Read the model definition and answer for the solid it produces. Units are mm, in the model's axes. Face numbers are marked on the shaded views. A direction names the side the tool comes from. Coordinates: 2 decimals unless noted, no trailing zeros. Order: outer loops, then holes, each group sorted by start corner. A loop starts at its lowest first (then second) coordinate and runs counter-clockwise, first axis right, second up. Notation, with made-up numbers: M -5,-29.75 L 42,-29.75 A22 cw 42,-12.75 Z; hole C 43.5,49 d6. An arc over 180 degrees is marked long. One line per question, with ' | ' between items. Start each with the question number.
1) Find section A-A, the plane z = 20. Write down the section's boundary in (x, y), plus the area to 3 significant figures.
2) Find section B-B, the plane x = 136. Write down the section's boundary in (y, z), plus the area to 3 significant figures.
3) A tool of negligible diameter and unlimited length cuts with its end or side. For the marked faces 1 and 2, from which of +Z, -Z, +X, -X, +Y, -Y can it reach the whole face along a straight path? Write none if from no direction.
4) Given P1, Ø5, axis at x = 72.5, y = 251.5, coming from the +Z side; P2, Ø5, axis at x = 79, z = 17, coming from the -Y side; P3, Ø5.5, axis at x = 76.2, z = 88.9, coming from the -Y side, each flat-ended and moving along its own axis, determine where each tip first touches the part or whether it passes through.
5) Consider probe 1 along Y at (x, z) = (77.5, 151); probe 2 along Z at (x, y) = (76, 8). Determine where each line is inside the solid, lowest interval first.
6) Find section C-C, the plane y = 323.5. Write down the section's boundary in (x, z), plus the area to 3 significant figures.
7) Find section D-D, the plane z = 122. Write down the section's boundary in (x, y), plus the area to 3 significant figures.
8) The mould has two halves that part along Y. Classify the marked faces 3, 4 and 5: +Y half, -Y half, draft (parallel to the pull), parting line (faces both ways), or undercut.
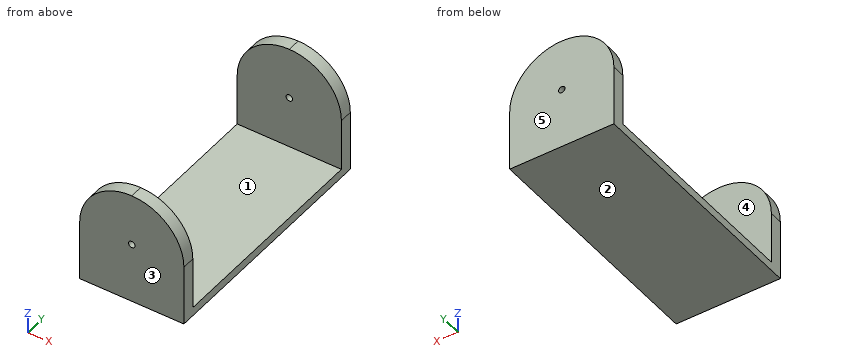
from build123d import *

# Parameters (mm, degrees)
F0_W     = 19.05
F0_H     = 152.4
F0_H_2   = 12.7
F0_W_2   = 317.5
F1_DEPTH = 152.4
F2_R     = 4.7625
F3_DEPTH = 406.4
F4_R     = 76.19999


# Not quite as in the source:
# - a fillet or chamfer is up to 0.001 mm smaller than in the source, because OpenCascade refuses the exact size


with BuildPart() as f1:
    # F0 (on Right) → F1 (new body)
    with BuildSketch(Plane.YZ):
        with Locations((9.525, 88.9)):
            Rectangle(F0_W, F0_H)
        with Locations((9.525, 6.35)):
            Rectangle(F0_W, F0_H_2)
        with Locations((177.8, 6.35)):
            Rectangle(F0_W_2, F0_H_2)
        with Locations((346.075, 88.9)):
            Rectangle(F0_W, F0_H)
        with Locations((346.075, 6.35)):
            Rectangle(F0_W, F0_H_2)
    extrude(amount=F1_DEPTH)

    # F2 (on Front) → F3 (cut)
    with BuildSketch(Plane.XZ):
        with Locations((76.2, 88.9)):
            Circle(F2_R)
    extrude(amount=-F3_DEPTH, mode=Mode.SUBTRACT)

    # F4 (radius 76.2 in the source; OpenCascade refuses exactly that, so slightly less here)
    f4_edges = [f1.edges().sort_by_distance(p)[0] for p in [
        (152.4, 346.075, 165.1),
        (152.4, 9.525, 165.1),
        (0, 9.525, 165.1),
        (0, 346.075, 165.1),
    ]]
    fillet(f4_edges, radius=F4_R)


solid = f1.part
Report:
1) outline: M 0,0 L 152.4,0 L 152.4,19.05 L 0,19.05 Z; M 0,336.55 L 152.4,336.55 L 152.4,355.6 L 0,355.6 Z | area: 5,810 mm^2
2) outline: M 0,0 L 355.6,0 L 355.6,136.13 L 336.55,136.13 L 336.55,12.7 L 19.05,12.7 L 19.05,136.13 L 0,136.13 Z | area: 9,220 mm^2
3) face 1: +Z, +X, -X | face 2: -Z, +X, -X, +Y, -Y
4) P1: stops at z = 12.7 | P2: stops at y = 0 | P3: passes through
5) probe 1: y = 0 to 19.05, 336.55 to 355.6 | probe 2: z = 0 to 84.14, 93.66 to 165.1
6) outline: M 0,0 L 152.4,0 L 152.4,12.7 L 0,12.7 Z | area: 1,940 mm^2
7) outline: M 7.56,0 L 144.84,0 L 144.84,19.05 L 7.56,19.05 Z; M 7.56,336.55 L 144.84,336.55 L 144.84,355.6 L 7.56,355.6 Z | area: 5,230 mm^2
8) face 3: -Y half | face 4: undercut | face 5: +Y half
